Check sheet for the modelled part. Datum: model origin and axes. Units: mm. A direction names the side the tool comes from. Coordinates: 2 decimals unless noted, no trailing zeros. Loops run counter-clockwise (first coordinate to the right, second up) from the corner with the lowest first, then second, coordinate; pieces in that order, holes last. Notation, with made-up numbers: (-16.75, 19) -> (31.25, 19) arc R20 ccw to (31.25, 56) -> close; hole circle Ø4 at (-29.75, 11). An arc over 180 degrees is marked (long way). Use one line per item in the form item = value.
from build123d import *

# Parameters (mm, degrees)
SKETCH1_W           = 23
SKETCH1_H           = 18.5
BOSS_EXTRUDE1_DEPTH = 1
FILLET1_R           = 1
BOSS_EXTRUDE2_START = 1.6
BOSS_EXTRUDE2_DEPTH = 1.6
BOSS_EXTRUDE3_DEPTH = 17.5
BOSS_EXTRUDE4_DEPTH = 11.5
FILLET2_R           = 6
SKETCH5_R           = 1.5
CUT_EXTRUDE1_DEPTH  = 9
SKETCH6_R           = 1.85
CUT_EXTRUDE3_DEPTH  = 3


with BuildPart() as part:
    # Sketch1 → Boss-Extrude1 (new body)
    with BuildSketch(Plane(origin=(0, 0, 0), x_dir=(1, 0, 0), z_dir=(0, 1, 0))):
        Rectangle(SKETCH1_W, SKETCH1_H)
    extrude(amount=BOSS_EXTRUDE1_DEPTH)

    # Fillet1
    fillet1_edges = [part.edges().sort_by_distance(p)[0] for p in [
        (11.5, 0.5, 9.25),
        (-11.5, 0.5, 9.25),
        (-11.5, 0.5, -9.25),
        (11.5, 0.5, -9.25),
    ]]
    fillet(fillet1_edges, radius=FILLET1_R)

    # Sketch2 → Boss-Extrude2 (add)
    with BuildSketch(Plane(origin=(0, 1, 0), x_dir=(1, 0, 0), z_dir=(0, 1, 0)).offset(BOSS_EXTRUDE2_START)):
        with BuildLine():
            Line((10.5, 9.25), (-10.5, 9.25))
            ThreePointArc((-10.5, 9.25), (-11.207106781, 8.957106781), (-11.5, 8.25))
            Line((-11.5, 8.25), (-11.5, -8.25))
            ThreePointArc((-11.5, -8.25), (-11.207106781, -8.957106781), (-10.5, -9.25))
            Line((-10.5, -9.25), (10.5, -9.25))
            ThreePointArc((10.5, -9.25), (11.207106781, -8.957106781), (11.5, -8.25))
            Line((11.5, -8.25), (11.5, 8.25))
            ThreePointArc((11.5, 8.25), (11.207106781, 8.957106781), (10.5, 9.25))
        make_face()
        with BuildLine():
            Line((9.25, 8.325), (-9.25, 8.325))
            ThreePointArc((-9.25, 8.325), (-10.098528137, 7.973528137), (-10.45, 7.125))
            Line((-10.45, 7.125), (-10.45, -7.125))
            ThreePointArc((-10.45, -7.125), (-10.098528137, -7.973528137), (-9.25, -8.325))
            Line((-9.25, -8.325), (9.25, -8.325))
            ThreePointArc((9.25, -8.325), (10.098528137, -7.973528137), (10.45, -7.125))
            Line((10.45, -7.125), (10.45, 7.125))
            ThreePointArc((10.45, 7.125), (10.098528137, 7.973528137), (9.25, 8.325))
        make_face(mode=Mode.SUBTRACT)
    extrude(amount=-BOSS_EXTRUDE2_DEPTH)

    # Sketch3 → Boss-Extrude3 (add)
    with BuildSketch(Plane(origin=(0, 0, 0), x_dir=(0, 0, -1), z_dir=(1, 0, 0))):
        Polygon((-2.824998215, -0.434236645), (-2.824998215, 0), (2.825004114, 0), (2.825004114, -0.52086856), (2.825004485, -2.050001378), (5.054655907, -2.050000837), (5.054655907, -3.096446609), (2.301102516, -5.85), (-2.297621726, -5.85), (-5.054652336, -2.959512633), (-5.054652336, -2.05), (-2.824998215, -2.05), align=None)
    extrude(amount=-BOSS_EXTRUDE3_DEPTH)

    # Sketch4 → Boss-Extrude4 (add)
    with BuildSketch(Plane(origin=(0, 0, 0), x_dir=(0, 0, -1), z_dir=(1, 0, 0))):
        Polygon((-2.824998215, -2.05), (2.825004485, -2.050001378), (2.825004114, 0), (-2.824998215, 0), align=None)
    extrude(amount=BOSS_EXTRUDE4_DEPTH)

    # Fillet2
    # the kernel refuses this fillet: 6 mm, written as the material it takes off along each edge
    with BuildSketch(Plane(origin=(0, -5.85, -16.256387574), x_dir=(0, 1, 0), z_dir=(0, 0, 1))) as fillet2_piece_1:
        with BuildLine():
            CenterArc((6, 5.582114023), FILLET2_R, 180, 68.489804657)
            Line((0, 5.582114023), (-0.12, 5.582114023))
            Line((-0.12, 5.582114023), (-0.12, 0))
            Line((-0.12, 0), (0, -0.12))
            ThreePointArc((0, -0.12), (1.899999655, -0.12), (3.755999297, -0.11164228))
            Line((3.755999297, -0.11164228), (3.799999311, 0))
        make_face()
    extrude(amount=32.509294358, mode=Mode.SUBTRACT)

    # Sketch5 → Cut-Extrude1 (cut)
    with BuildSketch(Plane(origin=(0, 0, 0), x_dir=(1, 0, 0), z_dir=(0, 1, 0))):
        with Locations(Location((-14.5, 0, 0), (0, 0, 270))):
            Circle(SKETCH5_R)
    extrude(amount=-CUT_EXTRUDE1_DEPTH, mode=Mode.SUBTRACT)

    # Sketch6 → Cut-Extrude3 (cut)
    with BuildSketch(Plane.XZ.offset(5.85)):
        with Locations(Location((-14.5, 0, 0), (0, 0, 270))):
            Circle(SKETCH6_R)
    extrude(amount=-CUT_EXTRUDE3_DEPTH, mode=Mode.SUBTRACT)


solid = part.part
(1) Mould release check, pull along X, two halves, no side actions. Record for faces 6 (the cylindrical face through (10.11, 1.81, -7.96)), 7 (the flat face through (0, 2, -8.325)), 8 (the cylindrical face through (-11.199, 1.318, -8.965)), 9 (the flat face through (-9, -2.05, 4)): +X half, -X half, draft (parallel to the pull), parting line (faces both ways), or undercut.
Established:
face_6 = undercut
face_7 = undercut
face_8 = -X half
face_9 = draft
(2) Scan lines: line 1 along X through (y, z) = (1.5, 4); line 2 along X through (y, z) = (-4.85, 0); line 3 along Y through (x, z) = (4.5, -6). Record each from-to range of solid material in increasing order.
Established:
line_1 = -11.5 to -10.45, 10.45 to 11.5
line_2 = -17.5 to -16.35, -12.65 to -2.27
line_3 = 0 to 1
(3) Section check B-B, the plane z = 1. Record the boundary of the cut face in (x, y).
Established:
outline = (-17.5, -5.85) -> (-16.06, -5.85) -> (-16.06, -2.85) -> (-15.62, -2.85) -> (-15.62, 0) -> (-17.5, 0) -> close; (-13.38, -2.85) -> (-12.94, -2.85) -> (-12.94, -5.85) -> (-5.58, -5.85) arc R6 ccw to (0, -2.05) -> (11.5, -2.05) -> (11.5, 2.6) -> (10.45, 2.6) -> (10.45, 1) -> (-10.45, 1) -> (-10.45, 2.6) -> (-11.5, 2.6) -> (-11.5, 0) -> (-13.38, 0) -> close
(4) Tool access check on faces 1 (the flat face through (-8.6, -2.6, -5.055)), 2 (the flat face through (0, 0, 6)), 3 (the flat face through (-13, 0, 1)), 4 (the flat face through (-9, -2.05, -4)), 5 (the flat face through (10.45, 2, 0)). Record the directions out of +Z, -Z, +X, -X, +Y, -Y that give a thin tool (end or side, any length) a straight path to the whole face; none if there is none.
Established:
face_1 = -Z, +X, -X, -Y
face_2 = +Z, +X, -X
face_3 = +Z, -Z, -X, +Y
face_4 = -Z, +X, -X
face_5 = +Y
(5) Go/stop test with flat-tipped pins: P1, Ø0.6, axis at x = -0.5, y = -1, coming from the +Z side (3 decimals); P2, Ø0.6, axis at x = 6.5, y = -0.5, coming from the -Z side (3 decimals); P3, Ø0.7, axis at x = -4.5, z = -4, coming from the +Y side; P4, Ø1, axis at x = -14.5, z = -0.5, coming from the -Y side. Record where each tip stops, or that it passes through.
Established:
P1 = 2.825
P2 = -2.825
P3 = 1
P4 = through
(6) Section check C-C, the plane y = 0.5. Record the boundary of the cut face in (x, z), plus the area to 3 significant figures.
Established:
outline = (-11.5, -8.25) arc R1 ccw to (-10.5, -9.25) -> (10.5, -9.25) arc R1 ccw to (11.5, -8.25) -> (11.5, 8.25) arc R1 ccw to (10.5, 9.25) -> (-10.5, 9.25) arc R1 ccw to (-11.5, 8.25) -> close
area = 425 mm²
(7) Section check A-A, the plane x = -14.5. Record the boundary of the cut face in (y, z) (3 decimals), plus the area to 3 significant figures.
Established:
outline = (-5.85, -2.301) -> (-3.096, -5.055) -> (-2.05, -5.055) -> (-2.05, -2.825) -> (-0.521, -2.825) -> (0, -2.825) -> (0, -1.5) -> (-2.85, -1.5) -> (-2.85, -1.85) -> (-5.85, -1.85) -> close; (-5.85, 1.85) -> (-2.85, 1.85) -> (-2.85, 1.5) -> (0, 1.5) -> (0, 2.825) -> (-2.05, 2.825) -> (-2.05, 5.055) -> (-2.96, 5.055) -> (-5.85, 2.298) -> close
area = 22.6 mm²
(8) Section check D-D, the plane x = 4.25. Record the boundary of the cut face in (y, z) (3 decimals).
Established:
outline = (-2.05, -2.825) -> (0, -2.825) -> (0, -9.25) -> (2.6, -9.25) -> (2.6, -8.325) -> (1, -8.325) -> (1, 8.325) -> (2.6, 8.325) -> (2.6, 9.25) -> (0, 9.25) -> (0, 2.825) -> (-2.05, 2.825) -> close
